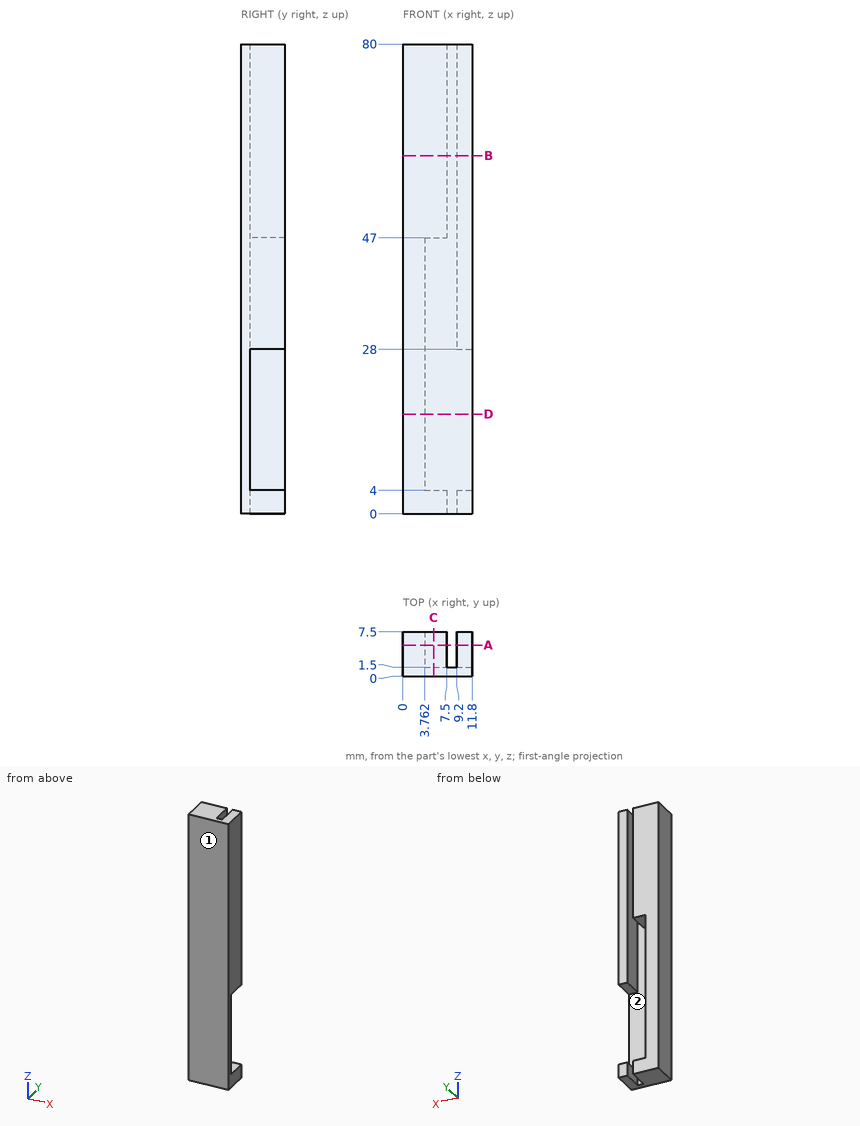
Study the drawing (mm; zero at the part's minimum x, y, z) and answer. Coordinates: 2 decimals unless noted, no trailing zeros. Write each loop counter-clockwise with the first axis right and the second up, starting at its lowest first coordinate (ties: lowest second). Pieces come first, ordered by that corner, then holes. Notation, with made-up numbers: M 47.5,-27.75 L 96.5,-27.75 A25 cw 96.5,5.25 Z; hole C 55.25,31 d2. An arc over 180 degrees is marked long. Write each question's results on one line, items separated by ' | '.
Item 1: The part is cut by section D-D on z = 17. Determine the outline of the cut face in (x, y), and give its area (3 significant figures).
Answer below:
outline: M 0,0 L 11.8,0 L 11.8,1.5 L 3.76,1.5 L 3.76,7.5 L 0,7.5 Z | area: 40.3 mm2
Item 2: The part is cut by section A-A on y = 5.25. Determine the outline of the cut face in (x, z), and give its area (3 significant figures).
Answer below:
outline: M 0,0 L 7.5,0 L 7.5,4 L 3.76,4 L 3.76,47 L 7.5,47 L 7.5,80 L 0,80 Z; M 9.2,0 L 11.8,0 L 11.8,4 L 9.2,4 Z; M 9.2,28 L 11.8,28 L 11.8,80 L 9.2,80 Z | area: 585 mm2
Item 3: The part is cut by section B-B on z = 61. Determine the outline of the cut face in (x, y).
Answer below:
outline: M 0,0 L 11.8,0 L 11.8,7.5 L 9.2,7.5 L 9.2,1.5 L 7.5,1.5 L 7.5,7.5 L 0,7.5 Z
Item 4: For a pull along X with two mould halves and no side action, classify the marked faces 1 and 2 as released by +X, released by -X, zero draft, split by the parting line, or undercut.
Answer below:
face 1: zero draft | face 2: undercut
Item 5: The part is cut by section C-C on x = 5.25. Determine the outline of the cut face in (y, z), and give its area (3 significant figures).
Answer below:
outline: M 0,0 L 7.5,0 L 7.5,4 L 1.5,4 L 1.5,47 L 7.5,47 L 7.5,80 L 0,80 Z | area: 342 mm2
Item 6: Given P1, Ø2.5, axis at x = 6.5, z = 35, coming from the +Y side, flat-ended and moving along its own axis, determine where the tip first touches the part or whether it passes through.
Answer below:
P1: y = 1.5
Item 7: Consider probe 1 along X at (y, z) = (5.25, 30); probe 2 along Z at (x, y) = (5.25, 5.5); probe 3 along X at (y, z) = (4, 54). Determine where each line is inside the solid, lowest interval first. Write a range as [from, to].
Answer below:
probe 1: [0, 3.76], [9.2, 11.8] | probe 2: [0, 4], [47, 80] | probe 3: [0, 7.5], [9.2, 11.8]
